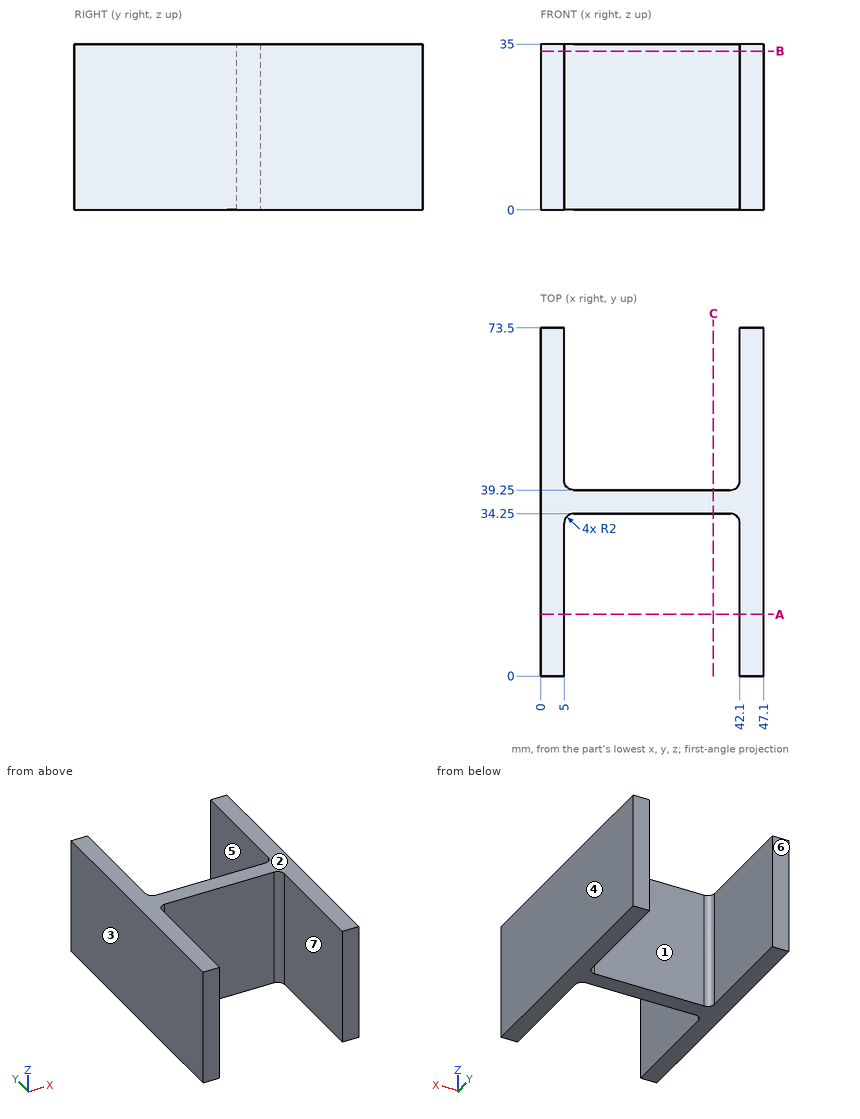
The drawing under review shows one solid part. Ordinate dimensions are in mm from its lowest x, y, z. A direction names the side the tool comes from. Coordinates: 2 decimals unless noted, no trailing zeros. Write each loop counter-clockwise with the first axis right and the second up, starting at its lowest first coordinate (ties: lowest second). Pieces come first, ordered by that corner, then holes. Notation, with made-up numbers: (-29, -27) - (24, -27) arc R18 ccw to (24, -7) - close; hole circle Ø9 at (-24, 53). An arc over 180 degrees is marked (long way). Use one line per item in the form item = value.
Q1. Consider section C-C (x = 36.5). Write out the cut boundary in (y, z).
Taken from the geometry:
outline = (34.25, 0) - (39.25, 0) - (39.25, 35) - (34.25, 35) - close
Q2. Machinability: for the marked faces 5, 6 and 7, which of the approach directions +Z, -Z, +X, -X, +Y, -Y give a long, thin tool a straight path to every point of the face, cutting with its end or side? Answer none if there is none.
Taken from the geometry:
face_5 = +Z, -Z, +Y
face_6 = +Z, -Z, +X, -X, +Y
face_7 = +Z, -Z, -Y
Q3. The part is to be moulded in two halves that separate along X. For the marked faces 1, 2, 3 and 4, say which applies: +X half, -X half, draft (parallel to the pull), parting line (faces both ways), or undercut.
Taken from the geometry:
face_1 = undercut
face_2 = draft
face_3 = -X half
face_4 = +X half
Q4. Insertion check: pin 1 Ø10 at (x, z) = (16, 13) entering from -Y; pin 2 Ø3 at (x, z) = (23.5, 4) entering from +Y. Each pin has a flat end and moves straight along its axis. Give the tip position at first contact, or say it passes through.
Taken from the geometry:
pin_1 = 34.25
pin_2 = 39.25
Q5. For probe 1 along X at (y, z) = (57, 30); probe 2 along Y at (x, z) = (32.5, 17.5); probe 3 along X at (y, z) = (39.5, 4.5), list the stretches that pass through material, from the lowest coordinate up.
Taken from the geometry:
probe_1 = 0 to 5, 42.1 to 47.1
probe_2 = 34.25 to 39.25
probe_3 = 0 to 6.03, 41.07 to 47.1
Q6. Consider section B-B (z = 33.5). Write out the cut boundary in (x, y).
Taken from the geometry:
outline = (0, 0) - (5, 0) - (5, 32.25) arc R2 cw to (7, 34.25) - (40.1, 34.25) arc R2 cw to (42.1, 32.25) - (42.1, 0) - (47.1, 0) - (47.1, 73.5) - (42.1, 73.5) - (42.1, 41.25) arc R2 cw to (40.1, 39.25) - (7, 39.25) arc R2 cw to (5, 41.25) - (5, 73.5) - (0, 73.5) - close
Q7. Consider section A-A (y = 13). Write out the cut boundary in (x, z).
Taken from the geometry:
outline = (0, 0) - (5, 0) - (5, 35) - (0, 35) - close; (42.1, 0) - (47.1, 0) - (47.1, 35) - (42.1, 35) - close
